Here's how the part is built. I have some questions about the finished solid (model axes, mm). A direction names the side the tool comes from. Round coordinates to 2 decimals unless told otherwise and drop trailing zeros. Order: outer loops, then holes, each group sorted by start corner. A loop starts at its lowest first (then second) coordinate and runs counter-clockwise, first axis right, second up. Notation, with made-up numbers: (37, 37.5) - (84, 37.5) arc R11 cw to (84, 50.5) - close; hole circle Ø1 at (3.25, 46.25). An arc over 180 degrees is marked (long way). One line per item, written item: value.
from build123d import *

# Parameters (mm, degrees)
BOSS_EXTRUDE1_DEPTH      = 0.1905
BOSS_EXTRUDE1_DEPTH_BACK = 0.1905


with BuildPart() as part:
    # Sketch1 → Boss-Extrude1 (new body, two sides)
    with BuildSketch(Plane.XY) as boss_extrude1_sk:
        with BuildLine():
            Line((-1.690782151, -2.92852059), (-0.725045158, -1.255815051))
            ThreePointArc((-0.725045158, -1.255815051), (-0.696082706, -1.089842323), (-0.781097204, -0.944383376))
            ThreePointArc((-0.781097204, -0.944383376), (-1.061357434, -0.612775), (-1.208408596, -0.204258333))
            ThreePointArc((-1.208408596, -0.204258333), (-1.291872491, -0.057904145), (-1.450090316, 0))
            Line((-1.450090316, 0), (-2.210471848, 0))
            ThreePointArc((-2.210471848, 0), (-2.471887729, 0.120306814), (-2.55054444, 0.397119231))
            ThreePointArc((-2.55054444, 0.397119231), (-2.235449712, 1.29063752), (-1.619187526, 2.010276693))
            ThreePointArc((-1.619187526, 2.010276693), (-1.340132599, 2.080564158), (-1.105235924, 1.914324775))
            Line((-1.105235924, 1.914324775), (-0.725045158, 1.255815051))
            ThreePointArc((-0.725045158, 1.255815051), (-0.595789785, 1.147746468), (-0.427311393, 1.148641709))
            ThreePointArc((-0.427311393, 1.148641709), (0, 1.22555), (0.427311393, 1.148641709))
            ThreePointArc((0.427311393, 1.148641709), (0.595789785, 1.147746468), (0.725045158, 1.255815051))
            Line((0.725045158, 1.255815051), (1.105235924, 1.914324775))
            ThreePointArc((1.105235924, 1.914324775), (1.340132631, 2.080564164), (1.619187578, 2.010276651))
            ThreePointArc((1.619187578, 2.010276651), (2.235449717, 1.290637512), (2.550544433, 0.397119278))
            ThreePointArc((2.550544433, 0.397119278), (2.471887745, 0.120306832), (2.210471848, 0))
            Line((2.210471848, 0), (1.450090316, 0))
            ThreePointArc((1.450090316, 0), (1.291872491, -0.057904145), (1.208408596, -0.204258333))
            ThreePointArc((1.208408596, -0.204258333), (1.061357434, -0.612775), (0.781097204, -0.944383376))
            ThreePointArc((0.781097204, -0.944383376), (0.696082706, -1.089842323), (0.725045158, -1.255815051))
            Line((0.725045158, -1.255815051), (1.690782151, -2.92852059))
            ThreePointArc((1.690782151, -2.92852059), (2.042375748, -3.177738803), (2.460517356, -3.073405821))
            ThreePointArc((2.460517356, -3.073405821), (0, 3.937), (-2.460517356, -3.073405821))
            ThreePointArc((-2.460517356, -3.073405821), (-2.042375748, -3.177738803), (-1.690782151, -2.92852059))
        make_face()
    extrude(amount=BOSS_EXTRUDE1_DEPTH)
    extrude(boss_extrude1_sk.sketch, amount=-BOSS_EXTRUDE1_DEPTH_BACK)


solid = part.part
Q1. If we section it at C-C, the plane z = -0.05: Please give me the cut outline in (x, y).
Results list:
outline: (-2.55, 0.4) arc R2.58 cw to (-1.62, 2.01) arc R0.34 cw to (-1.11, 1.91) - (-0.73, 1.26) arc R0.25 ccw to (-0.43, 1.15) arc R1.23 cw to (0.43, 1.15) arc R0.25 ccw to (0.73, 1.26) - (1.11, 1.91) arc R0.34 cw to (1.62, 2.01) arc R2.58 cw to (2.55, 0.4) arc R0.34 cw to (2.21, 0) - (1.45, 0) arc R0.25 ccw to (1.21, -0.2) arc R1.23 cw to (0.78, -0.94) arc R0.25 ccw to (0.73, -1.26) - (1.69, -2.93) arc R0.52 ccw to (2.46, -3.07) arc R3.94 ccw (long way) to (-2.46, -3.07) arc R0.52 ccw to (-1.69, -2.93) - (-0.73, -1.26) arc R0.25 ccw to (-0.78, -0.94) arc R1.23 cw to (-1.21, -0.2) arc R0.25 ccw to (-1.45, 0) - (-2.21, 0) arc R0.34 cw to start
Q2. If we section it at B-B, the plane x = 1: Please give me the cut outline in (y, z), then the cut area to 3 significant figures.
Results list:
outline: (-1.73, -0.19) - (-0.71, -0.19) - (-0.71, 0.19) - (-1.73, 0.19) - close; (1.73, -0.19) - (3.81, -0.19) - (3.81, 0.19) - (1.73, 0.19) - close
area: 1.18 mm²
Q3. If I drill on line 1 along X through (y, z) = (2, 0); line 2 along Y through (x, z) = (-2.25, 0); line 3 along Y through (x, z) = (-1, 0.1), over which ranges is the centre line in solid material (lowest first)?
Results list:
line 1: -3.39 to -1.63, -1.18 to 1.18, 1.63 to 3.39
line 2: -3.17 to 0, 1.27 to 3.23
line 3: -1.73 to -0.71, 1.73 to 3.81
Q4. If we section it at D-D, the plane x = 0: Please give me the cut outline in (y, z).
Results list:
outline: (1.23, -0.19) - (3.94, -0.19) - (3.94, 0.19) - (1.23, 0.19) - close
Q5. If we section it at A-A, the plane y = -2.25: Please give me the cut outline in (x, z), then the cut area to 3 significant figures.
Results list:
outline: (-3.23, -0.19) - (-1.3, -0.19) - (-1.3, 0.19) - (-3.23, 0.19) - close; (1.3, -0.19) - (3.23, -0.19) - (3.23, 0.19) - (1.3, 0.19) - close
area: 1.47 mm²
Q6. We'd pull the mould along X, two halves only. Please class faces 1 (the cylindrical face through (0.136, 3.935, 0.003)), 2 (the flat face through (1.2, -2.08, 0)), 3 (the flat face through (0, 2, 0.19)): released by +X, released by -X, zero draft, split by the parting line, or undercut.
Results list:
face 1: split by the parting line
face 2: undercut
face 3: zero draft
Q7. Which directions (+Z, -Z, +X, -X, +Y, -Y) give clear straight access to the entire face, cutting with the end or side of a thin tool? Please do faces 4 (the cylindrical face through (-2.24, 1.28, 0)), 5 (the flat face through (-1.215, -2.104, 0.003)), 6 (the flat face through (0, 2, -0.19)).
Results list:
face 4: +Z, -Z
face 5: +Z, -Z, -Y
face 6: -Z, +X, -X, +Y, -Y
